```python
from build123d import *

# Parameters (mm, degrees)
SKETCH_1_W          = 27
SKETCH_1_H          = 10
SKETCH_1_R          = 1.6
EXTRUDE_1_DEPTH     = 3
CUT_EXTRUDE_1_DEPTH = 3.5
FILLET_1_R          = 1.5
CHAMFER_1_SIZE      = 0.5


with BuildPart() as part:
    # Эскиз1 → Бобышка-Вытянуть1 (new body)
    with BuildSketch(Plane(origin=(0, 0, 0), x_dir=(1, 0, 0), z_dir=(0, 1, 0))):
        Rectangle(SKETCH_1_W, SKETCH_1_H)
        with Locations(Location((-8.5, 0, 0), (0, 0, 270))):
            Circle(SKETCH_1_R, mode=Mode.SUBTRACT)
        with Locations(Location((8.5, 0, 0), (0, 0, 270))):
            Circle(SKETCH_1_R, mode=Mode.SUBTRACT)
    extrude(amount=EXTRUDE_1_DEPTH)

    # Эскиз2 → Вырез-Вытянуть1 (cut, symmetric)
    with BuildSketch(Plane(origin=(0, 0, 0), x_dir=(0, 0, -1), z_dir=(1, 0, 0))):
        with BuildLine():
            ThreePointArc((-3.494902022, 0.318181818), (-3.701518997, 0.086176097), (-4, 0))
            Line((-4, 0), (-2, 0))
            ThreePointArc((-2, 0), (-2.298481003, 0.086176097), (-2.505097978, 0.318181818))
            ThreePointArc((-2.505097978, 0.318181818), (-2.56176419, 0.46533442), (-2.594594195, 0.619565217))
            ThreePointArc((-2.594594195, 0.619565217), (-2.644405657, 0.712771412), (-2.743312728, 0.75))
            Line((-2.743312728, 0.75), (-3.256687272, 0.75))
            ThreePointArc((-3.256687272, 0.75), (-3.355594343, 0.712771412), (-3.405405805, 0.619565217))
            ThreePointArc((-3.405405805, 0.619565217), (-3.43823581, 0.46533442), (-3.494902022, 0.318181818))
        make_face()
        with BuildLine():
            ThreePointArc((-4.594594195, 0.619565217), (-4.644405657, 0.712771412), (-4.743312728, 0.75))
            Line((-4.743312728, 0.75), (-5, 0.75))
            Line((-5, 0.75), (-5, 0))
            Line((-5, 0), (-4, 0))
            ThreePointArc((-4, 0), (-4.298481003, 0.086176097), (-4.505097978, 0.318181818))
            ThreePointArc((-4.505097978, 0.318181818), (-4.56176419, 0.46533442), (-4.594594195, 0.619565217))
        make_face()
        with BuildLine():
            ThreePointArc((-1.494902022, 0.318181818), (-1.701518997, 0.086176097), (-2, 0))
            Line((-2, 0), (0, 0))
            ThreePointArc((0, 0), (-0.298481003, 0.086176097), (-0.505097978, 0.318181818))
            ThreePointArc((-0.505097978, 0.318181818), (-0.56176419, 0.46533442), (-0.594594195, 0.619565217))
            ThreePointArc((-0.594594195, 0.619565217), (-0.644405657, 0.712771412), (-0.743312728, 0.75))
            Line((-0.743312728, 0.75), (-1.256687272, 0.75))
            ThreePointArc((-1.256687272, 0.75), (-1.355594343, 0.712771412), (-1.405405805, 0.619565217))
            ThreePointArc((-1.405405805, 0.619565217), (-1.43823581, 0.46533442), (-1.494902022, 0.318181818))
        make_face()
        with BuildLine():
            ThreePointArc((0.505097978, 0.318181818), (0.298481003, 0.086176097), (0, 0))
            Line((0, 0), (2, 0))
            ThreePointArc((2, 0), (1.701518997, 0.086176097), (1.494902022, 0.318181818))
            ThreePointArc((1.494902022, 0.318181818), (1.43823581, 0.46533442), (1.405405805, 0.619565217))
            ThreePointArc((1.405405805, 0.619565217), (1.355594343, 0.712771412), (1.256687272, 0.75))
            Line((1.256687272, 0.75), (0.743312728, 0.75))
            ThreePointArc((0.743312728, 0.75), (0.644405657, 0.712771412), (0.594594195, 0.619565217))
            ThreePointArc((0.594594195, 0.619565217), (0.56176419, 0.46533442), (0.505097978, 0.318181818))
        make_face()
        with BuildLine():
            ThreePointArc((2.505097978, 0.318181818), (2.298481003, 0.086176097), (2, 0))
            Line((2, 0), (4, 0))
            ThreePointArc((4, 0), (3.701518997, 0.086176097), (3.494902022, 0.318181818))
            ThreePointArc((3.494902022, 0.318181818), (3.43823581, 0.46533442), (3.405405805, 0.619565217))
            ThreePointArc((3.405405805, 0.619565217), (3.355594343, 0.712771412), (3.256687272, 0.75))
            Line((3.256687272, 0.75), (2.743312728, 0.75))
            ThreePointArc((2.743312728, 0.75), (2.644405657, 0.712771412), (2.594594195, 0.619565217))
            ThreePointArc((2.594594195, 0.619565217), (2.56176419, 0.46533442), (2.505097978, 0.318181818))
        make_face()
        with BuildLine():
            ThreePointArc((4.505097978, 0.318181818), (4.298481003, 0.086176097), (4, 0))
            Line((4, 0), (5, 0))
            Line((5, 0), (5, 0.75))
            Line((5, 0.75), (4.743312728, 0.75))
            ThreePointArc((4.743312728, 0.75), (4.644405657, 0.712771412), (4.594594195, 0.619565217))
            ThreePointArc((4.594594195, 0.619565217), (4.56176419, 0.46533442), (4.505097978, 0.318181818))
        make_face()
    extrude(amount=CUT_EXTRUDE_1_DEPTH, both=True, mode=Mode.SUBTRACT)

    # Скругление1
    fillet_1_edges = [part.edges().sort_by_distance(p)[0] for p in [
        (-13.5, 3, 0),
        (0, 3, 5),
        (13.5, 3, 0),
        (0, 3, -5),
        (13.5, 1.5, 5),
        (-13.5, 1.5, 5),
        (-13.5, 1.5, -5),
        (13.5, 1.5, -5),
    ]]
    fillet(fillet_1_edges, radius=FILLET_1_R)

    # Фаска1
    chamfer_1_edges = [part.edges().sort_by_distance(p)[0] for p in [
        (-8.5, 0, -1.6),
        (-8.5, 3, -1.6),
        (8.5, 0, -1.6),
        (8.5, 3, -1.6),
    ]]
    chamfer(chamfer_1_edges, length=CHAMFER_1_SIZE)


solid = part.part
```
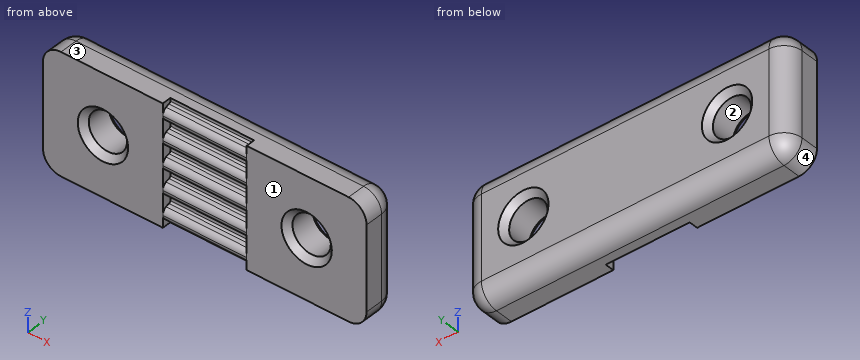
Build history of the part. All positions in model axes, mm. Face numbers are marked on the shaded views. Give positions to 0.01 mm unless a question says otherwise; leave off trailing zeros. Loops run counter-clockwise (first coordinate to the right, second up) from the corner with the lowest first, then second, coordinate; pieces in that order, holes last. Notation, with made-up numbers: (74.25, 88.25) -> (114.25, 88.25) arc R11 ccw to (114.25, 107.25) -> close; hole circle Ø9 at (67, 84). An arc over 180 degrees is marked (long way). One line per question, with ' | ' between items.
Q1. Drill centre lines: line 1 along X through (y, z) = (1.55, 0); line 2 along X through (y, z) = (1.2, -0.75); line 3 along Y through (x, z) = (-3, 1.25). Where is each one in solid material? Low to high. Write a range as [from, to].
Filled sheet:
line 1: x = [-13.5, -10.1], [-6.9, 6.9], [10.1, 13.5] | line 2: x = [-13.5, -9.91], [-7.09, 7.09], [9.91, 13.5] | line 3: y = [0.75, 3]
Q2. Pull direction Z, two halves, no side cores. Call the marked faces 1, 2, 3 and 4: pulls with the +Z half, pulls with the -Z half, needs draft (parallel to the pull), parting line crosses it, or undercut.
Filled sheet:
face 1: needs draft | face 2: undercut | face 3: pulls with the +Z half | face 4: pulls with the -Z half
Q3. Cut at A-A, the plane y = 1.2. Write the cut outline in (x, z).
Filled sheet:
outline: (-13.5, -3.5) arc R1.5 ccw to (-12, -5) -> (12, -5) arc R1.5 ccw to (13.5, -3.5) -> (13.5, 3.5) arc R1.5 ccw to (12, 5) -> (-12, 5) arc R1.5 ccw to (-13.5, 3.5) -> close; hole circle Ø3.2 at (-8.5, 0); hole circle Ø3.2 at (8.5, 0)
Q4. Cut at C-C, the plane z = -1. Count the separate pieces of the cut face and the enclosed holes in it, plus the area to 3 significant figures.
Filled sheet:
separate pieces: 3 | enclosed holes: 0 | area: 58.6 mm²
Q5. Cut at B-B, the plane x = -8.5. Write the cut outline in (y, z).
Filled sheet:
outline: (0, -5) -> (1.5, -5) arc R1.5 ccw to (3, -3.5) -> (3, -2.1) -> (2.5, -1.6) -> (0.5, -1.6) -> (0, -2.1) -> close; (0, 2.1) -> (0.5, 1.6) -> (2.5, 1.6) -> (3, 2.1) -> (3, 3.5) arc R1.5 ccw to (1.5, 5) -> (0, 5) -> close
Q6. Drop flat-ended pins along their axis: pin 1 (4 mm diameter, centred on x = -9, z = 1.5, fed in from -Y); pin 2 (1.5 mm diameter, centred on x = -4, y = 2.5, fed in from -Z); pin 3 (0.6 mm diameter, centred on y = 0.5, z = -4.5, fed in from +X). Give the stop position or say it passes through.
Filled sheet:
pin 1: stops at y = 0 | pin 2: stops at z = -4.98 | pin 3: stops at x = 13.33
